Verification items for the finished model (mm, model axes). Face numbers are marked on the shaded views. A direction names the side the tool comes from. Give positions to 0.01 mm unless a question says otherwise; leave off trailing zeros. Loops run counter-clockwise (first coordinate to the right, second up) from the corner with the lowest first, then second, coordinate; pieces in that order, holes last. Notation, with made-up numbers: (46, 75) - (57, 75) arc R11 cw to (57, 80) - close; hole circle Ø8 at (85, -6.75). An arc over 180 degrees is marked (long way). One line per item, written item: value. Start each with the question number.
1. Gauge pin test, flat ends, axial feed: pin 1 (6 mm diameter, centred on y = 70.5, z = 165, fed in from -X); pin 2 (6 mm diameter, centred on x = -38, z = 104, fed in from -Y); pin 3 (10.5 mm diameter, centred on x = 78.5, z = 160.5, fed in from -Y); pin 4 (2.5 mm diameter, centred on x = -84, y = 5, fed in from -Z). Record the tip position at first contact, or that the pin passes through.
2. Sectioned sample at B-B (x = 7.5). Record the cut outline in (y, z), plus the area to 3 significant figures.
3. Scan lines: L1, parallel to X at y = 76, z = 85; L2, parallel to X at y = 14, z = 90; L3, parallel to X at y = 29.5, z = 63. Record each from-to range of solid material in increasing order. Write a range as [from, to].
4. Sectioned sample at A-A (z = 130). Record the cut outline in (x, y).
5. Mould release check, pull along X, two halves, no side actions. Record for the marked faces 1, 2 and 3: pulls with the +X half, pulls with the -X half, needs draft (parallel to the pull), parting line crosses it, or undercut.
6. Sectioned sample at C-C (x = -18.75). Record the cut outline in (y, z), plus the area to 3 significant figures.
7. Access from +Z, -Z, +X, -X, +Y, -Y to the whole of each face (thin tool, end or side, straight path). Record for the marked faces 4 and 5.
8. Sectioned sample at D-D (z = 61.5). Record the cut outline in (x, y), plus the area to 3 significant figures.
from build123d import *

# Parameters (mm, degrees)
SKETCH_1_W           = 175
SKETCH_1_H           = 160
EXTRUDE_1_DEPTH      = 193
FILLET_8_R           = 40
SHELL_2_T            = -5
SKETCH_9_W           = 95
SKETCH_9_H           = 80
CUT_EXTRUDE_3_DEPTH  = 10
SKETCH_10_R          = 35
CUT_EXTRUDE_4_DEPTH  = 160
SKETCH_12_W          = 40
SKETCH_12_H          = 60
CUT_EXTRUDE_5_DEPTH  = 20
CUT_EXTRUDE_6_DEPTH  = 80
SKETCH_15_R          = 2.5
CUT_EXTRUDE_7_DEPTH  = 5
SKETCH_17_R          = 2.5
CUT_EXTRUDE_9_DEPTH  = 5
CUT_EXTRUDE_10_DEPTH = 2
SKETCH_23_R          = 2.5
CUT_EXTRUDE_13_DEPTH = 5


with BuildPart() as part:
    # 草圖1 → 填料-伸長1 (new body)
    with BuildSketch(Plane.XY):
        Rectangle(SKETCH_1_W, SKETCH_1_H)
    extrude(amount=EXTRUDE_1_DEPTH)

    # 圓角8
    fillet_8_edges = [part.edges().sort_by_distance(p)[0] for p in [
        (-87.5, 0, 193),
        (0, -80, 193),
        (87.5, 0, 193),
        (0, 80, 193),
    ]]
    fillet(fillet_8_edges, radius=FILLET_8_R)

    # 薄殼2
    shell_2_openings = [part.faces().sort_by_distance(p)[0] for p in [
        (0, 0, 0),
    ]]
    offset(amount=SHELL_2_T, openings=shell_2_openings)

    # 草圖9 → 除料-伸長3 (cut)
    with BuildSketch(Plane.XY.offset(193)):
        Rectangle(SKETCH_9_W, SKETCH_9_H)
    extrude(amount=-CUT_EXTRUDE_3_DEPTH, mode=Mode.SUBTRACT)

    # 草圖10 → 除料-伸長4 (cut)
    with BuildSketch(Plane(origin=(0, 80, 0), x_dir=(1, 0, 0), z_dir=(0, 1, 0))):
        with Locations((-18.75, -12.103072957)):
            Circle(SKETCH_10_R)
    extrude(amount=-CUT_EXTRUDE_4_DEPTH, mode=Mode.SUBTRACT)

    # 草圖12 → 除料-伸長5 (cut)
    with BuildSketch(Plane(origin=(90, 0, 0), x_dir=(0, 0, -1), z_dir=(1, 0, 0))):
        with Locations((-155.457670656, 0)):
            Rectangle(SKETCH_12_W, SKETCH_12_H)
    extrude(amount=-CUT_EXTRUDE_5_DEPTH, mode=Mode.SUBTRACT)

    # 草圖4 → 除料-伸長6 (cut)
    with BuildSketch(Plane(origin=(0, 0, 0), x_dir=(1, 0, 0), z_dir=(0, 1, 0))):
        Polygon((0, -200), (-165, -200), (-165, 0), (110, 0), (110, -200), align=None)
    extrude(amount=-CUT_EXTRUDE_6_DEPTH, mode=Mode.SUBTRACT)

    # 草圖15 → 除料-伸長7 (cut)
    with BuildSketch(Plane(origin=(0, 80, 0), x_dir=(1, 0, 0), z_dir=(0, 1, 0))):
        with Locations(Location((7.5, -85, 0), (0, 0, 270))):
            Circle(SKETCH_15_R)
        with Locations(Location((-7.5, -85, 0), (0, 0, 270))):
            Circle(SKETCH_15_R)
    extrude(amount=-CUT_EXTRUDE_7_DEPTH, mode=Mode.SUBTRACT)

    # 草圖17 → 除料-伸長9 (cut)
    with BuildSketch(Plane.ZY.offset(87.5)):
        with Locations((130, 40)):
            Circle(SKETCH_17_R)
        with Locations((142.5, 40)):
            Circle(SKETCH_17_R)
        with Locations((70, 25)):
            Circle(SKETCH_17_R)
        with Locations((95, 25)):
            Circle(SKETCH_17_R)
        Polygon((65, 0), (65, -10), (85, -10), (85, 20), (65, 20), align=None)
    extrude(amount=-CUT_EXTRUDE_9_DEPTH, mode=Mode.SUBTRACT)

    # 草圖18 → 除料-伸長10 (cut)
    with BuildSketch(Plane(origin=(87.5, 0, 0), x_dir=(0, 0, -1), z_dir=(1, 0, 0))):
        with BuildLine():
            Line((-67.728835328, 0), (-89.728835328, 0))
            Line((-89.728835328, 0), (-89.62835003, 2.295574964))
            Line((-89.62835003, 2.295574964), (-89.76926499, 7.293588867))
            ThreePointArc((-89.76926499, 7.293588867), (-76.170437541, 35.347471494), (-48.437401965, 49.589212124))
            ThreePointArc((-48.437401965, 49.589212124), (-63.441387718, 26.87910562), (-67.728835328, 0))
        make_face()
    extrude(amount=-CUT_EXTRUDE_10_DEPTH, mode=Mode.SUBTRACT)

    # 草圖23 → 除料-伸長13 (cut)
    with BuildSketch(Plane(origin=(85.5, 0, 0), x_dir=(0, 0, -1), z_dir=(1, 0, 0))):
        with Locations((-84.69880751, 4.794581915)):
            Circle(SKETCH_23_R)
    extrude(amount=-CUT_EXTRUDE_13_DEPTH, mode=Mode.SUBTRACT)


solid = part.part
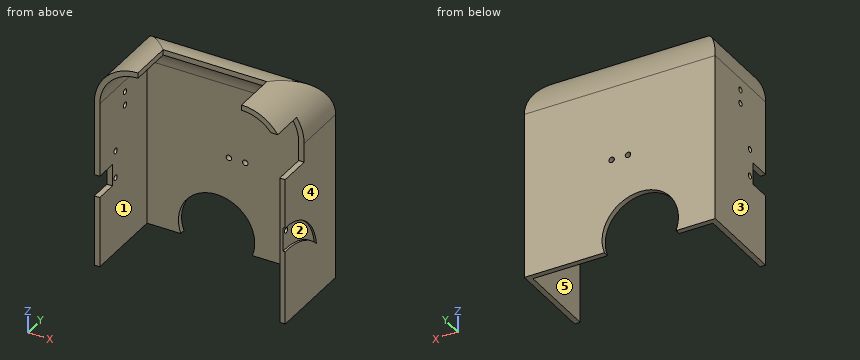
Results are:
1. pin 1: stops at x = -86.47
1. pin 2: stops at y = 75
1. pin 3: stops at y = 30
1. pin 4: stops at z = 0
2. outline: (40, 188) arc R35 cw to (75, 153) - (75, 87.5) - (80, 87.5) - (80, 153) arc R40 ccw to (40, 193) - close; (75, 35.25) - (80, 35.25) - (80, 82.5) - (75, 82.5) - close
2. area: 858 mm^2
3. L1: x = [-87.5, -10], [-5, 5], [10, 87.5]
3. L2: x = [-87.5, -82.5], [82.5, 87.5]
3. L3: x = [-87.5, -82.5], [82.5, 85.5]
4. outline: (-87.5, 0) - (-82.5, 0) - (-82.5, 37.5) - (-87.5, 37.5) - close; (-87.5, 42.5) - (-82.5, 42.5) - (-82.5, 75) - (82.5, 75) - (82.5, 0) - (87.5, 0) - (87.5, 80) - (-87.5, 80) - close
5. face 1: undercut
5. face 2: pulls with the +X half
5. face 3: pulls with the -X half
6. outline: (40, 188) arc R35 cw to (75, 153) - (75, 47.1) - (80, 47.1) - (80, 153) arc R40 ccw to (40, 193) - close
6. area: 824 mm^2
7. face 4: +Z, -Z, +X, +Y, -Y
7. face 5: -Z, -Y
8. outline: (-87.5, 0) - (-82.5, 0) - (-82.5, 75) - (82.5, 75) - (82.5, 0) - (87.5, 0) - (87.5, 31.36) - (85.5, 31.36) - (85.5, 45.68) - (87.5, 45.68) - (87.5, 80) - (-87.5, 80) - close
8. area: 1,600 mm^2
